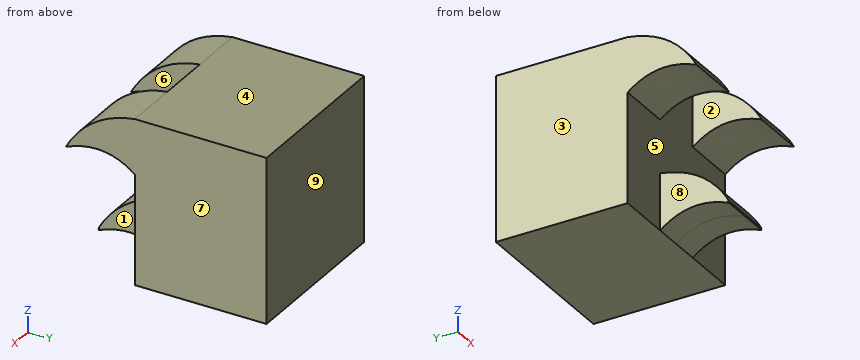
from build123d import *

# Parameters (mm, degrees)
SKETCH_1_W               = 15
SKETCH_1_H               = 15
EXTRUDE_1_DEPTH          = 6
EXTRUDE_2_DEPTH          = 2.5
PATTERN_START            = -7.5
PATTERN_SKETCH_2_DEPTH   = 5
PATTERN_START_2          = 2.5
PATTERN_SKETCH_2_2_DEPTH = 5
PATTERN_START_3          = -2.5
PATTERN_SKETCH_2_3_DEPTH = 5


# Read off the part's stored shape, not the designer's step: 스케치 패턴2
with BuildPart() as part:
    # 스케치1 → 보스-돌출1 (new, symmetric)
    with BuildSketch(Plane(origin=(0, 0, 0), x_dir=(1, 0, 0), z_dir=(0, 1, 0))):
        Rectangle(SKETCH_1_W, SKETCH_1_H)
    extrude(amount=EXTRUDE_1_DEPTH, both=True)

    # 스케치3 → 보스-돌출2 (add, symmetric)
    with BuildSketch(Plane(origin=(0, 0, 0), x_dir=(0, 0, -1), z_dir=(1, 0, 0))):
        with BuildLine():
            Line((2.5, -6), (7.5, -6))
            add(Edge.make_bspline(
                [(6.837946582, -12.278081575), (5.299376428, -8.730527415), (7.5, -6)],
                knots=[0, 0, 0, 1, 1, 1], degree=2))
            add(Edge.make_bspline(
                [(2.5, -6), (3.098107293, -10.225865232), (6.837946582, -12.278081575)],
                knots=[0, 0, 0, 1, 1, 1], degree=2))
        make_face()
    extrude(amount=EXTRUDE_2_DEPTH, both=True)

    # 스케치 패턴2 outline → 스케치 패턴2 (add)
    with BuildSketch(Plane.YZ.offset(PATTERN_START)):
        with BuildLine():
            add(Edge.make_bspline(
                [(-12.278081575, 3.16045553), (-8.730527415, 4.699025684), (-6, 2.498402112)],
                knots=[0, 0, 0, 1, 1, 1], degree=2))
            Line((-6, 2.498402112), (-6, 7.498402112))
            add(Edge.make_bspline(
                [(-6, 7.498402112), (-10.225865232, 6.900294818), (-12.278081575, 3.16045553)],
                knots=[0, 0, 0, 1, 1, 1], degree=2))
        make_face()
    extrude(amount=PATTERN_SKETCH_2_DEPTH)

    # Pattern Sketch 2 2 outline → Pattern Sketch 2 2 (add)
    with BuildSketch(Plane.YZ.offset(PATTERN_START_2)):
        with BuildLine():
            add(Edge.make_bspline(
                [(-12.278081575, 3.16045553), (-8.730527415, 4.699025684), (-6, 2.498402112)],
                knots=[0, 0, 0, 1, 1, 1], degree=2))
            Line((-6, 2.498402112), (-6, 7.498402112))
            add(Edge.make_bspline(
                [(-6, 7.498402112), (-10.225865232, 6.900294818), (-12.278081575, 3.16045553)],
                knots=[0, 0, 0, 1, 1, 1], degree=2))
        make_face()
    extrude(amount=PATTERN_SKETCH_2_2_DEPTH)

    # Pattern Sketch 2 3 outline → Pattern Sketch 2 3 (add)
    with BuildSketch(Plane.YZ.offset(PATTERN_START_3)):
        with BuildLine():
            add(Edge.make_bspline(
                [(-6, -2.341597888), (-10.225865232, -2.939705182), (-12.278081575, -6.67954447)],
                knots=[0, 0, 0, 1, 1, 1], degree=2))
            add(Edge.make_bspline(
                [(-12.278081575, -6.67954447), (-12.219236087, -6.65402325), (-12.160615404, -6.629530866)],
                knots=[0, 0, 0, 0.016587622, 0.016587622, 0.016587622], degree=2))
            add(Edge.make_bspline(
                [(-6, -2.5), (-10.106703233, -3.081241715), (-12.160615404, -6.629530866)],
                knots=[0, 0, 0, 0.971801751, 0.971801751, 0.971801751], degree=2))
            Line((-6, -2.5), (-6, -2.341597888))
        make_face()
    extrude(amount=PATTERN_SKETCH_2_3_DEPTH)


solid = part.part
Model file for the job. Use its own axes, mm. Face numbers are marked on the shaded views. A direction names the side the tool comes from. Coordinates: 2 decimals unless noted, no trailing zeros. Loops run counter-clockwise (first coordinate to the right, second up) from the corner with the lowest first, then second, coordinate; pieces in that order, holes last. Notation, with made-up numbers: (22.25, 10.25) -> (78.25, 10.25) arc R27 ccw to (78.25, 28.25) -> close; hole circle Ø11 at (61, -40). An arc over 180 degrees is marked (long way). Use one line per item in the form item = value. Start each with the question number.
(1) Cut at A-A on z = 1.5. Give the cut face in (x, y).
(2) Tool access for the marked faces 1, 2, 3, 4 and 5: list every direction of +Z, -Z, +X, -X, +Y, -Y with a clear straight run to the whole face (end or side of a thin tool).
(3) Pull direction X, two halves, no side cores. Call the marked faces 6, 7, 8 and 9: pulls with the +X half, pulls with the -X half, needs draft (parallel to the pull), parting line crosses it, or undercut.
(4) Cut at B-B on y = -10.75. Give the number of separate pieces and of enclosed holes in the cut face, and give its area (3 significant figures).
(5) Probe probe 1 along Y at (x, z) = (-2.5, 1.25); probe 2 along Z at (x, y) = (-2.75, -8); probe 3 along Y at (x, z) = (7, 5.5). List the from-to ranges inside material, lowest first. Write a range as from..to.
(6) Flat gauge pins, fed straight in: pin 1 (7.5 mm diameter, centred on x = -0.5, z = -1.5, fed in from -Y); pin 2 (2.5 mm diameter, centred on y = -8.5, z = -4, fed in from +X); pin 3 (1 mm diameter, centred on y = -8.5, z = 3.5, fed in from -X); pin 4 (2.5 mm diameter, centred on y = -9, z = -4.5, fed in from -X). Where does each tip first touch, or does it go through?
Values:
q1.outline = (-7.5, -6) -> (7.5, -6) -> (7.5, 6) -> (-7.5, 6) -> close
q2.face_1 = -Z, +X, -Y
q2.face_2 = +Z, -Y
q2.face_3 = +Z, -Z, -X, +Y, -Y
q2.face_4 = +Z, +X, -X, +Y, -Y
q2.face_5 = -Y
q3.face_6 = undercut
q3.face_7 = pulls with the +X half
q3.face_8 = pulls with the -X half
q3.face_9 = needs draft
q4.separate_pieces = 3
q4.enclosed_holes = 0
q4.area = 24.3 mm2
q5.probe_1 = -6..6
q5.probe_2 = 3.58..6.99
q5.probe_3 = -10.46..6
q6.pin_1 = -11.32
q6.pin_2 = 2.5
q6.pin_3 = -7.5
q6.pin_4 = -2.5
